Verification items for the finished model (mm, model axes). A direction names the side the tool comes from. Coordinates: 2 decimals unless noted, no trailing zeros. Order: outer loops, then holes, each group sorted by start corner. A loop starts at its lowest first (then second) coordinate and runs counter-clockwise, first axis right, second up. Notation, with made-up numbers: M -2.75,61 L 4.25,61 A10 ccw 4.25,78 Z; hole C 49.5,-7.5 d2. An arc over 180 degrees is marked long. Return JSON: item names as keys, results as strings. Group by question number.
Q1. Section check C-C, the plane x = 23. Count the separate pieces of the cut face and the enclosed holes in it, then the cut area to 3 significant figures.
Q2. Go/stop test with flat-tipped pins: pin 1 Ø3.5 at (x, z) = (-29.5, 1) entering from -Y; pin 2 Ø4 at (x, z) = (-12, 16) entering from +Y; pin 3 Ø2 at (x, z) = (8.5, 6) entering from -Y. Record where each tip stops, or that it passes through.
Q3. Access from +Z, -Z, +X, -X, +Y, -Y to the whole of each face (thin tool, end or side, straight path). Record for faces 4 (the face through (-5, 13, 2)), 5 (the face through (-32.04, -0.21, 10.6)), 6 (the face through (-19.25, 21, 1)).
Q4. Section check D-D, the plane y = -18. Enter the section's corners in (x, z), then the cut area to 3 significant figures.
Q5. Section check A-A, the plane x = 3.5. Enter the section's corners in (y, z).
Q6. Section check B-B, the plane y = -2. Enter the section's corners in (x, z), then the cut area to 3 significant figures.
Q7. Thickness scan on probe 1 along Y at (x, z) = (-9.5, 2.35); probe 2 along Y at (x, z) = (23, 0.85); probe 3 along X at (y, z) = (-0.5, 2.75). Record the ranges inside material, lowest first.
Q8. Mould release check, pull along Y, two halves, no side actions. Record for faces 1 (the face through (-20.11, -17.3, 1.52)), 2 (the face through (31.74, 11.79, 1.52)), 3 (the face through (-30.61, -0.23, 9.79)): pulls with the +Y half, pulls with the -Y half, needs draft (parallel to the pull), parting line crosses it, or undercut.
from build123d import *

# Parameters (mm, degrees)
SKETCH1_W           = 74.8
SKETCH1_H           = 32.8
BOSS_EXTRUDE1_DEPTH = 3
CUT_EXTRUDE1_DEPTH  = 3
SKETCH3_R           = 1.75
CUT_EXTRUDE2_DEPTH  = 3
SKETCH4_W           = 48.5
SKETCH4_H           = 18
CUT_EXTRUDE3_DEPTH  = 3
SKETCH5_W           = 57.5
SKETCH5_H           = 21
SKETCH5_W_2         = 48.5
SKETCH5_H_2         = 18
BOSS_EXTRUDE3_DEPTH = 15
CUT_EXTRUDE11_START = -10.6
CUT_EXTRUDE11_DEPTH = 21
CHAMFER1_SIZE       = 15
CHAMFER1_SIZE2      = 3
CHAMFER2_SIZE       = 3
CHAMFER2_SIZE2      = 15
SKETCH18_W          = 54.5
SKETCH18_H          = 18
SKETCH18_W_2        = 53
SKETCH18_H_2        = 17
BOSS_EXTRUDE6_DEPTH = 3
SKETCH12_W          = 29.5
SKETCH12_H          = 10
BOSS_EXTRUDE5_DEPTH = 3
SKETCH13_R          = 2.1
CUT_EXTRUDE9_DEPTH  = 3
FILLET2_R           = 3
FILLET3_R           = 3
FILLET4_R           = 4
FILLET5_R           = 3
FILLET11_R          = 2
CHAMFER11_SIZE      = 2.383507185
CHAMFER11_SIZE_2    = 2
CUT_EXTRUDE12_DEPTH = 2
CUT_EXTRUDE13_DEPTH = 2
SKETCH21_R          = 4
CUT_EXTRUDE14_DEPTH = 2


# Read off the part's stored shape, not the designer's step: Cut-Extrude11
with BuildPart() as part:
    # Sketch1 → Boss-Extrude1 (new body)
    with BuildSketch(Plane.XY):
        Rectangle(SKETCH1_W, SKETCH1_H)
    extrude(amount=BOSS_EXTRUDE1_DEPTH)

    # Sketch2 → Cut-Extrude1 (cut)
    with BuildSketch(Plane.XY.offset(3)):
        Polygon((37.4, 16.4), (26.4, 16.4), (37.4, 6.9), align=None)
        Polygon((37.4, -16.4), (37.4, -6.9), (26.4, -16.4), align=None)
    extrude(amount=-CUT_EXTRUDE1_DEPTH, mode=Mode.SUBTRACT)

    # Sketch3 → Cut-Extrude2 (cut)
    with BuildSketch(Plane.XY.offset(3)):
        with Locations((-33, 12)):
            Circle(SKETCH3_R)
        with Locations((-33, -12)):
            Circle(SKETCH3_R)
        with Locations((23, -12)):
            Circle(SKETCH3_R)
        with Locations((23, 12)):
            Circle(SKETCH3_R)
    extrude(amount=-CUT_EXTRUDE2_DEPTH, mode=Mode.SUBTRACT)

    # Sketch4 → Cut-Extrude3 (cut)
    with BuildSketch(Plane.XY.offset(3)):
        with Locations((-5, -0.1)):
            Rectangle(SKETCH4_W, SKETCH4_H)
    extrude(amount=-CUT_EXTRUDE3_DEPTH, mode=Mode.SUBTRACT)

    # Sketch5 → Boss-Extrude3 (add)
    with BuildSketch(Plane.XY.offset(3)):
        with Locations((-5, -0.1)):
            Rectangle(SKETCH5_W, SKETCH5_H)
        with Locations((-5, -0.1)):
            Rectangle(SKETCH5_W_2, SKETCH5_H_2, mode=Mode.SUBTRACT)
    extrude(amount=BOSS_EXTRUDE3_DEPTH)

    # Cut-Extrude11 outline → Cut-Extrude11 (cut)
    with BuildSketch(Plane(origin=(0, 0, 0), x_dir=(1, 0, 0), z_dir=(0, 1, 0)).offset(CUT_EXTRUDE11_START)):
        Polygon((-33.75, -3), (-33.75, -18), (-30.286977133, -3), align=None)
        Polygon((23.75, -3), (20.286977133, -3), (23.75, -18), align=None)
    extrude(amount=CUT_EXTRUDE11_DEPTH, mode=Mode.SUBTRACT)

    # Chamfer1
    chamfer1_edges = [part.edges().sort_by_distance(p)[0] for p in [
        (19.25, -0.1, 18),
    ]]
    chamfer1_side = [part.faces().sort_by_distance(p)[0] for p in [
        (19.25, -0.1, 9),
    ]]
    chamfer(chamfer1_edges, length=CHAMFER1_SIZE, length2=CHAMFER1_SIZE2, reference=chamfer1_side[0])

    # Chamfer2
    chamfer2_edges = [part.edges().sort_by_distance(p)[0] for p in [
        (-29.25, -0.1, 18),
    ]]
    chamfer2_side = [part.faces().sort_by_distance(p)[0] for p in [
        (-3.5, 9.512147858, 18),
    ]]
    chamfer(chamfer2_edges, length=CHAMFER2_SIZE, length2=CHAMFER2_SIZE2, reference=chamfer2_side[0])

    # Sketch18 → Boss-Extrude6 (add)
    with BuildSketch(Plane.XY.offset(18)):
        with Locations((-5, -0.1)):
            Rectangle(SKETCH18_W, SKETCH18_H)
        with Locations((-5, -0.1)):
            Rectangle(SKETCH18_W_2, SKETCH18_H_2, mode=Mode.SUBTRACT)
    extrude(amount=-BOSS_EXTRUDE6_DEPTH)

    # Sketch12 → Boss-Extrude5 (add)
    with BuildSketch(Plane(origin=(0, 0, 0), x_dir=(-1, 0, 0), z_dir=(0, 0, -1))):
        with Locations((4.5, 21.4)):
            Rectangle(SKETCH12_W, SKETCH12_H)
        with Locations((4.5, -21.4)):
            Rectangle(SKETCH12_W, SKETCH12_H)
    extrude(amount=-BOSS_EXTRUDE5_DEPTH)

    # Sketch13 → Cut-Extrude9 (cut)
    with BuildSketch(Plane(origin=(0, 0, 0), x_dir=(-1, 0, 0), z_dir=(0, 0, -1))):
        with Locations((-0.5, 22.4)):
            Circle(SKETCH13_R)
        with Locations((9.5, 22.4)):
            Circle(SKETCH13_R)
        with Locations((-0.5, -22.4)):
            Circle(SKETCH13_R)
        with Locations((9.5, -22.4)):
            Circle(SKETCH13_R)
    extrude(amount=-CUT_EXTRUDE9_DEPTH, mode=Mode.SUBTRACT)

    # Fillet2
    fillet2_edges = [part.edges().sort_by_distance(p)[0] for p in [
        (22.018488567, 10.4, 10.5),
        (22.018488567, -10.6, 10.5),
        (-32.018488566, -10.6, 10.5),
        (-32.018488566, 10.4, 10.5),
    ]]
    fillet(fillet2_edges, radius=FILLET2_R)

    # Fillet3
    fillet3_edges = [part.edges().sort_by_distance(p)[0] for p in [
        (37.4, 6.9, 1.5),
        (26.4, 16.4, 1.5),
        (26.4, -16.4, 1.5),
        (37.4, -6.9, 1.5),
        (-37.4, -16.4, 1.5),
        (-37.4, 16.4, 1.5),
    ]]
    fillet(fillet3_edges, radius=FILLET3_R)

    # Fillet4
    fillet4_edges = [part.edges().sort_by_distance(p)[0] for p in [
        (-19.25, 26.4, 1.5),
        (10.25, 26.4, 1.5),
        (10.25, -26.4, 1.5),
        (-19.25, -26.4, 1.5),
    ]]
    fillet(fillet4_edges, radius=FILLET4_R)

    # Fillet5
    fillet5_edges = [part.edges().sort_by_distance(p)[0] for p in [
        (-19.25, 16.4, 1.5),
        (10.25, 16.4, 1.5),
        (10.25, -16.4, 1.5),
        (-19.25, -16.4, 1.5),
    ]]
    fillet(fillet5_edges, radius=FILLET5_R)

    # Fillet11
    fillet11_edges = [part.edges().sort_by_distance(p)[0] for p in [
        (21.5, 8.4, 16.5),
        (-31.5, 8.4, 16.5),
        (-31.5, -8.6, 16.5),
        (21.5, -8.6, 16.5),
    ]]
    fillet(fillet11_edges, radius=FILLET11_R)

    # Chamfer11
    # the kernel refuses this chamfer: 2.383507185, 2 mm, written as the material it takes off along each edge
    with BuildSketch(Plane(origin=(-31.5, -6.6, 15), x_dir=(0.024939322090233706, 0, 0.9996889667359941), z_dir=(0, 1, 0))) as chamfer11_piece_1_section:
        Polygon((CHAMFER11_SIZE * 0.999688966815, -CHAMFER11_SIZE * 0.0249393220922), (-CHAMFER11_SIZE_2 * 0.0249393220902, -CHAMFER11_SIZE_2 * 0.999688966736), (0, 0), align=None)
    chamfer11_piece_1 = extrude(amount=13, mode=Mode.PRIVATE)
    chamfer11_piece_1 = split(chamfer11_piece_1, bisect_by=Plane(origin=(-31.892473609, -0.1, 16.212368046), z_dir=(0.9805806756909202, 0, 0.196116135138184)), keep=Keep.TOP, mode=Mode.PRIVATE)
    add(chamfer11_piece_1, mode=Mode.SUBTRACT)
    with BuildSketch(Plane(origin=(19.5, -8.6, 15), x_dir=(0, 0.024939322090234427, 0.9996889667359941), z_dir=(-1, 0, 0))) as chamfer11_piece_2_section:
        Polygon((CHAMFER11_SIZE * 0.999688966815, -CHAMFER11_SIZE * 0.0249393220922), (-CHAMFER11_SIZE_2 * 0.0249393220902, -CHAMFER11_SIZE_2 * 0.999688966736), (0, 0), align=None)
    chamfer11_piece_2 = extrude(amount=49, mode=Mode.PRIVATE)
    chamfer11_piece_2 = split(chamfer11_piece_2, bisect_by=Plane(origin=(-5, -9.1, 16.074399324), z_dir=(0, 1, 0)), keep=Keep.TOP, mode=Mode.PRIVATE)
    add(chamfer11_piece_2, mode=Mode.SUBTRACT)
    with BuildSketch(Plane(origin=(-29.5, 8.4, 15), x_dir=(0, -0.024939322090234427, 0.9996889667359941), z_dir=(1, 0, 0))) as chamfer11_piece_3_section:
        Polygon((CHAMFER11_SIZE * 0.999688966815, -CHAMFER11_SIZE * 0.0249393220922), (-CHAMFER11_SIZE_2 * 0.0249393220902, -CHAMFER11_SIZE_2 * 0.999688966736), (0, 0), align=None)
    chamfer11_piece_3 = extrude(amount=49, mode=Mode.PRIVATE)
    chamfer11_piece_3 = split(chamfer11_piece_3, bisect_by=Plane(origin=(-5, 8.9, 16.074399324), z_dir=(0, -1, 0)), keep=Keep.TOP, mode=Mode.PRIVATE)
    add(chamfer11_piece_3, mode=Mode.SUBTRACT)
    with BuildSketch(Plane(origin=(21.5, 6.4, 15), x_dir=(-0.024939322090233706, 0, 0.9996889667359941), z_dir=(0, -1, 0))) as chamfer11_piece_4_section:
        Polygon((CHAMFER11_SIZE * 0.999688966815, -CHAMFER11_SIZE * 0.0249393220922), (-CHAMFER11_SIZE_2 * 0.0249393220902, -CHAMFER11_SIZE_2 * 0.999688966736), (0, 0), align=None)
    chamfer11_piece_4 = extrude(amount=13, mode=Mode.PRIVATE)
    chamfer11_piece_4 = split(chamfer11_piece_4, bisect_by=Plane(origin=(21.892473609, -0.1, 16.212368046), z_dir=(-0.9805806756909202, 0, 0.19611613513818402)), keep=Keep.TOP, mode=Mode.PRIVATE)
    add(chamfer11_piece_4, mode=Mode.SUBTRACT)
    with BuildSketch(Plane(origin=(-29.5, -6.6, 15), x_dir=(-1, 0, 0), z_dir=(0, 1, 0))) as chamfer11_piece_5_section:
        Polygon((2, CHAMFER11_SIZE), (2 + CHAMFER11_SIZE_2, 0), (2, 0), align=None)
    chamfer11_piece_5 = revolve(axis=Axis((-29.5, -6.6, 15), (0, 0, 1)), revolution_arc=90, mode=Mode.PRIVATE)
    chamfer11_piece_5 = split(chamfer11_piece_5, bisect_by=Plane(origin=(-31.818510416, -8.221304707, 15.842552081), z_dir=(0.9805806756909202, 0, 0.196116135138184)), keep=Keep.TOP, mode=Mode.PRIVATE)
    chamfer11_piece_5 = split(chamfer11_piece_5, bisect_by=Plane(origin=(-30.957610473, -9.1, 16.014732069), z_dir=(0, 1, 0)), keep=Keep.TOP, mode=Mode.PRIVATE)
    add(chamfer11_piece_5, mode=Mode.SUBTRACT)
    with BuildSketch(Plane(origin=(19.5, -6.6, 15), x_dir=(0, -1, 0), z_dir=(-1, 0, 0))) as chamfer11_piece_6_section:
        Polygon((2, CHAMFER11_SIZE), (2 + CHAMFER11_SIZE_2, 0), (2, 0), align=None)
    chamfer11_piece_6 = revolve(axis=Axis((19.5, -6.6, 15), (0, 0, 1)), revolution_arc=90, mode=Mode.PRIVATE)
    chamfer11_piece_6 = split(chamfer11_piece_6, bisect_by=Plane(origin=(21.818510413, -8.221304708, 15.842552067), z_dir=(-0.9805806756909202, 0, 0.19611613513818402)), keep=Keep.TOP, mode=Mode.PRIVATE)
    chamfer11_piece_6 = split(chamfer11_piece_6, bisect_by=Plane(origin=(20.957610477, -9.1, 16.014732055), z_dir=(0, 1, 0)), keep=Keep.TOP, mode=Mode.PRIVATE)
    add(chamfer11_piece_6, mode=Mode.SUBTRACT)
    with BuildSketch(Plane(origin=(-29.5, 6.4, 15), x_dir=(0, 1, 0), z_dir=(1, 0, 0))) as chamfer11_piece_7_section:
        Polygon((2, CHAMFER11_SIZE), (2 + CHAMFER11_SIZE_2, 0), (2, 0), align=None)
    chamfer11_piece_7 = revolve(axis=Axis((-29.5, 6.4, 15), (0, 0, 1)), revolution_arc=90, mode=Mode.PRIVATE)
    chamfer11_piece_7 = split(chamfer11_piece_7, bisect_by=Plane(origin=(-30.957610477, 8.9, 16.014732055), z_dir=(0, -1, 0)), keep=Keep.TOP, mode=Mode.PRIVATE)
    chamfer11_piece_7 = split(chamfer11_piece_7, bisect_by=Plane(origin=(-31.818510413, 8.021304708, 15.842552067), z_dir=(0.9805806756909202, 0, 0.196116135138184)), keep=Keep.TOP, mode=Mode.PRIVATE)
    add(chamfer11_piece_7, mode=Mode.SUBTRACT)
    with BuildSketch(Plane(origin=(19.5, 6.4, 15), x_dir=(0, 1, 0), z_dir=(-1, 0, 0))) as chamfer11_piece_8_section:
        Polygon((2, -CHAMFER11_SIZE), (2 + CHAMFER11_SIZE_2, 0), (2, 0), align=None)
    chamfer11_piece_8 = revolve(axis=Axis((19.5, 6.4, 15), (0, 0, -1)), revolution_arc=90, mode=Mode.PRIVATE)
    chamfer11_piece_8 = split(chamfer11_piece_8, bisect_by=Plane(origin=(21.818510414, 8.021304708, 15.842552069), z_dir=(-0.9805806756909202, 0, 0.19611613513818402)), keep=Keep.TOP, mode=Mode.PRIVATE)
    chamfer11_piece_8 = split(chamfer11_piece_8, bisect_by=Plane(origin=(20.957610476, 8.9, 16.014732056), z_dir=(0, -1, 0)), keep=Keep.TOP, mode=Mode.PRIVATE)
    add(chamfer11_piece_8, mode=Mode.SUBTRACT)

    # Sketch19 → Cut-Extrude12 (cut)
    with BuildSketch(Plane(origin=(0, 0, 0), x_dir=(-1, 0, 0), z_dir=(0, 0, -1))):
        with BuildLine():
            Line((0, 14.4), (10, 14.4))
            ThreePointArc((10, 14.4), (11.25, 13.15), (10, 11.9))
            Line((10, 11.9), (0, 11.9))
            ThreePointArc((0, 11.9), (-1.25, 13.15), (0, 14.4))
        make_face()
    extrude(amount=-CUT_EXTRUDE12_DEPTH, mode=Mode.SUBTRACT)

    # Sketch20 → Cut-Extrude13 (cut)
    with BuildSketch(Plane(origin=(0, 0, 0), x_dir=(-1, 0, 0), z_dir=(0, 0, -1))):
        with BuildLine():
            Line((35.9, -1.15), (35.9, -7.15))
            ThreePointArc((35.9, -7.15), (34.65, -8.4), (33.4, -7.15))
            Line((33.4, -7.15), (33.4, -1.15))
            ThreePointArc((33.4, -1.15), (34.65, 0.1), (35.9, -1.15))
        make_face()
    extrude(amount=-CUT_EXTRUDE13_DEPTH, mode=Mode.SUBTRACT)

    # Sketch21 → Cut-Extrude14 (cut)
    with BuildSketch(Plane(origin=(0, 0, 0), x_dir=(-1, 0, 0), z_dir=(0, 0, -1))):
        with Locations((-28.5, 0)):
            Circle(SKETCH21_R)
    extrude(amount=-CUT_EXTRUDE14_DEPTH, mode=Mode.SUBTRACT)


solid = part.part
Numbers:
{
 "1": {"separate pieces": "4", "enclosed holes": "0", "area": "135 mm2"},
 "2": {"pin 1": "stops at y = -16.4", "pin 2": "stops at y = 10.4", "pin 3": "stops at y = -10.6"},
 "3": {"face 4": "-Z", "face 5": "-X, +Y, -Y", "face 6": "+Z, -Z, -X, +Y"},
 "4": {"outline": "M -19.6,0 L 10.6,0 L 10.6,3 L -19.6,3 Z", "area": "90.6 mm2"},
 "5": {"outline": "M -26.4,0 L -9.1,0 L -9.1,16.79 L -8.6,17.38 L -8.6,18 L -10.6,18 L -10.6,3 L -26.4,3 Z; M 8.4,17.38 L 8.9,16.79 L 8.9,0 L 26.4,0 L 26.4,3 L 10.4,3 L 10.4,18 L 8.4,18 Z"},
 "6": {"outline": "M -37.4,0 L -35.9,0 L -35.9,2 L -33.4,2 L -33.4,0 L -29.25,0 L -29.25,3 L -32.01,16.78 L -31.5,17.38 L -31.5,18 L -33.75,18 L -30.29,3 L -37.4,3 Z; M 19.25,0 L 25.04,0 L 25.04,2 L 31.96,2 L 31.96,0 L 37.4,0 L 37.4,3 L 20.29,3 L 23.75,18 L 21.5,18 L 21.5,17.38 L 22.01,16.78 L 19.25,3 Z", "area": "99.3 mm2"},
 "7": {"probe 1": "y = -26.4 to -24.5, -20.3 to -9.1, 8.9 to 20.3, 24.5 to 26.4", "probe 2": "y = -16.4 to -13.75, -10.25 to 10.25, 13.75 to 16.4", "probe 3": "x = -37.4 to -29.25, 19.25 to 37.4"},
 "8": {"face 1": "pulls with the -Y half", "face 2": "pulls with the +Y half", "face 3": "undercut"}
}
